Input: part model. Units: mm. Frame: model coordinates. Face numbers are marked on the shaded views. A direction names the side the tool comes from. Round coordinates to 2 decimals unless told otherwise and drop trailing zeros. Order: outer loops, then holes, each group sorted by start corner. A loop starts at its lowest first (then second) coordinate and runs counter-clockwise, first axis right, second up. Notation, with made-up numbers: (-11, 34.5) -> (23, 34.5) arc R22 ccw to (23, 43.5) -> close; hole circle Ø9 at (12.25, 16.25). An arc over 180 degrees is marked (long way). Use a Markdown table: item, result.
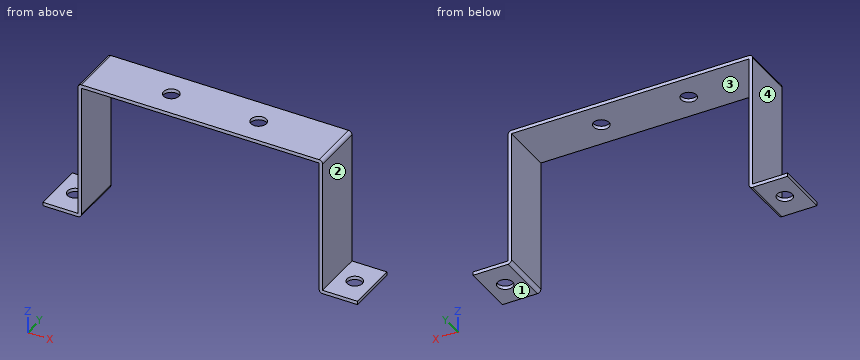
from build123d import *

# Parameters (mm, degrees)
F1_DEPTH = 30
F2_R     = 4.4
F3_R     = 4.4
F4_DEPTH = 25
F5_R     = 2
F6_R     = 2


# Not quite as in the source:
# - a feature names something its author has since deleted; it is built from what else it names


with BuildPart() as f1:
    # F0 (on Front) → F1 (new body)
    with BuildSketch(Plane.XZ):
        Polygon((90, -1), (90, 1), (70, 1), (70, 79), (-70, 79), (-70, 1), (-90, 1), (-90, -1), (-68, -1), (-68, 77), (68, 77), (68, -1), align=None)
    extrude(amount=F1_DEPTH)

    # F2 (on face) + F3 (on face) → F4 (cut)
    with BuildSketch(Plane.XY.offset(1)):
        with Locations((-80, -15)):
            Circle(F2_R)
        with Locations((80, -15)):
            Circle(F2_R)
    with BuildSketch(Plane.XY.offset(79)):
        with Locations((-25, -15)):
            Circle(F3_R)
        with Locations((25, -15)):
            Circle(F3_R)
    extrude(amount=-F4_DEPTH, mode=Mode.SUBTRACT)

    # F5
    f5_edges = [f1.edges().sort_by_distance(p)[0] for p in [
        (-70, -15, 79),
        (70, -15, 79),
    ]]
    fillet(f5_edges, radius=F5_R)

    # F6
    f6_edges = [f1.edges().sort_by_distance(p)[0] for p in [
        (68, -15, -1),
        (-68, -15, -1),
    ]]
    fillet(f6_edges, radius=F6_R)


solid = f1.part
1) Cut plane C-C on y = -26. Return loops of the section in (x, z), and give its area (3 significant figures).
Results found:
| item | result |
|---|---|
| outline | (-90, -1) -> (-70, -1) arc R2 ccw to (-68, 1) -> (-68, 77) -> (68, 77) -> (68, 1) arc R2 ccw to (70, -1) -> (90, -1) -> (90, 1) -> (70, 1) -> (70, 77) arc R2 ccw to (68, 79) -> (-68, 79) arc R2 ccw to (-70, 77) -> (-70, 1) -> (-90, 1) -> close |
| area | 669 mm² |
2) Cut plane B-B on x = 25. Return loops of the section in (y, z), and give its area (3 significant figures).
Results found:
| item | result |
|---|---|
| outline | (-30, 77) -> (-19.4, 77) -> (-19.4, 79) -> (-30, 79) -> close; (-10.6, 77) -> (0, 77) -> (0, 79) -> (-10.6, 79) -> close |
| area | 42.4 mm² |
3) Pin query (flat end, axial travel): pin 1 Ø11.5 at (x, y) = (80, -15) entering from -Z; pin 2 Ø5.5 at (x, y) = (-25, -15) entering from -Z; pin 3 Ø5 at (y, z) = (-8, 13.5) entering from -X; pin 4 Ø5 at (y, z) = (-7.5, 27) entering from +X. Return the tip coordinate at first contact, or that it passes through.
Results found:
| item | result |
|---|---|
| pin 1 | stops at z = -1 |
| pin 2 | passes through |
| pin 3 | stops at x = -70 |
| pin 4 | stops at x = 70 |
4) Cut plane A-A on z = 23.5. Return loops of the section in (x, y).
Results found:
| item | result |
|---|---|
| outline | (-70, -30) -> (-68, -30) -> (-68, 0) -> (-70, 0) -> close; (68, -30) -> (70, -30) -> (70, 0) -> (68, 0) -> close |
5) Set-up query: the marked faces 1, 2, 3 and 4. Return all of +Z, -Z, +X, -X, +Y, -Y with unobstructed straight access to the full face (end or side cutting, diameter ignored); none if empty.
Results found:
| item | result |
|---|---|
| face 1 | -Z, +X, -X, +Y, -Y |
| face 2 | +Z, +X, +Y, -Y |
| face 3 | -Z, +Y, -Y |
| face 4 | +Z, -X, +Y, -Y |
6) Line query: L1, parallel to X at y = -27.75, z = 56.5; L2, parallel to Y at x = -80, z = -0.55; L3, parallel to Z at x = 24, y = -21. Output: solid intervals per line, ascending. Write a range as [from, to].
Results found:
| item | result |
|---|---|
| L1 | x = [-70, -68], [68, 70] |
| L2 | y = [-30, -19.4], [-10.6, 0] |
| L3 | z = [77, 79] |
7) Cut plane D-D on x = 52. Return loops of the section in (y, z), and give its area (3 significant figures).
Results found:
| item | result |
|---|---|
| outline | (-30, 77) -> (0, 77) -> (0, 79) -> (-30, 79) -> close |
| area | 60.0 mm² |
